```python
from build123d import *
from build123d.topology import SkipClean

# Parameters (mm, degrees)
BOSS_EXTRUDE1_DEPTH    = 3
SKETCH1_R              = 2
BOSS_EXTRUDE1_2_DEPTH  = 3
BOSS_EXTRUDE2_DEPTH    = 3
M4_TAPPED_HOLE1_REACH  = 33.171
M4_TAPPED_HOLE1_BORE_R = 1.65


with BuildPart() as part:
    # Sketch1 → Boss-Extrude1 (new, symmetric)
    with BuildSketch(Plane.XY):
        with BuildLine():
            ThreePointArc((5.5, 0), (0, -5.5), (-5.5, 0))
            Line((-5.5, 0), (-12.42820323, -4))
            ThreePointArc((-12.42820323, -4), (0, -16.42820323), (12.42820323, -4))
            Line((12.42820323, -4), (5.5, 0))
        make_face()
    extrude(amount=BOSS_EXTRUDE1_DEPTH, both=True)



with BuildPart() as body_2:
    # Sketch1 → Boss-Extrude1 2 (new, symmetric)
    with BuildSketch(Plane.XY):
        with BuildLine():
            Line((-3.929058411, 8.75), (-5.402455316, 1.03125))
            ThreePointArc((-5.402455316, 1.03125), (0, 5.5), (5.402455316, 1.03125))
            Line((5.402455316, 1.03125), (3.929058411, 8.75))
            ThreePointArc((3.929058411, 8.75), (0, 12), (-3.929058411, 8.75))
        make_face()
        with Locations((0, 8)):
            Circle(SKETCH1_R, mode=Mode.SUBTRACT)
    extrude(amount=BOSS_EXTRUDE1_2_DEPTH, both=True)


with BuildPart() as part_1:
    with SkipClean():  # the faces are left unmerged after this step: merging them gives an invalid solid
        add(part.part)

        add(body_2.part)  # Boss-Extrude2 merges body 2
        # Sketch1<3> → Boss-Extrude2 (add, symmetric)
        with BuildSketch(Plane.XY):
            with BuildLine():
                ThreePointArc((-3.5, 0), (0, 3.5), (3.5, 0))
                Line((3.5, 0), (5.5, 0))
                ThreePointArc((5.5, 0), (5.475559526, 0.517926522), (5.402455316, 1.03125))
                ThreePointArc((5.402455316, 1.03125), (0, 5.5), (-5.402455316, 1.03125))
                ThreePointArc((-5.402455316, 1.03125), (-5.475559526, 0.517926522), (-5.5, 0))
                Line((-5.5, 0), (-3.5, 0))
            make_face()
            with BuildLine():
                Line((5.5, 0), (3.5, 0))
                ThreePointArc((3.5, 0), (0, -3.5), (-3.5, 0))
                Line((-3.5, 0), (-5.5, 0))
                ThreePointArc((-5.5, 0), (0, -5.5), (5.5, 0))
            make_face()
        extrude(amount=BOSS_EXTRUDE2_DEPTH, both=True)

    # M4 Tapped Hole1 bore → M4 Tapped Hole1 (cut, up to next)
    with BuildSketch(Plane(origin=(0, -16.42820323, 0), x_dir=(-1, 0, 0), z_dir=(0, -1, 0)), mode=Mode.PRIVATE) as m4_tapped_hole1_sk1:
        Circle(M4_TAPPED_HOLE1_BORE_R)
    m4_tapped_hole1_tool1 = extrude(m4_tapped_hole1_sk1.sketch, amount=-M4_TAPPED_HOLE1_REACH, mode=Mode.PRIVATE) & part_1.part
    add(m4_tapped_hole1_tool1.solids().sort_by_distance((0, -16.428203, 0))[0], mode=Mode.SUBTRACT)


solid = part_1.part
```
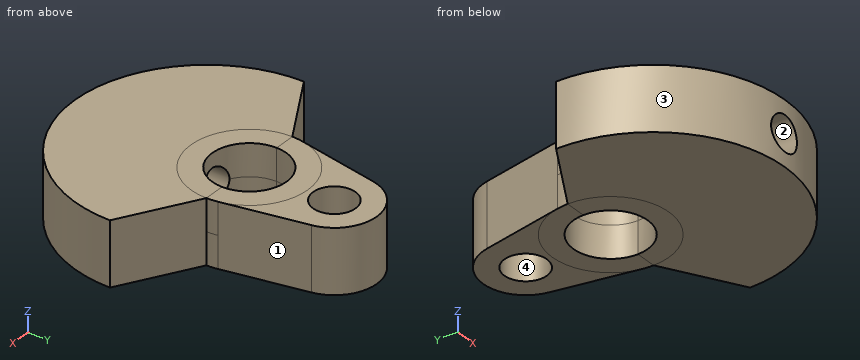
The listing builds one solid part. Answer for the finished solid, in the listing's coordinates (mm). Face numbers are marked on the shaded views. Give positions to 0.01 mm unless a question says otherwise; leave off trailing zeros. Order: outer loops, then holes, each group sorted by start corner. A loop starts at its lowest first (then second) coordinate and runs counter-clockwise, first axis right, second up. Notation, with made-up numbers: M -32.5,51.5 L -14.5,51.5 A30 ccw -14.5,83.5 Z; hole C 14,84 d9. An arc over 180 degrees is marked long. Put each result on its own line as item: value. Start each with the question number.
Item 1: For a pull along Y with two mould halves and no side action, classify the marked faces 1, 2, 3 and 4 as +Y half, -Y half, draft (parallel to the pull), parting line (faces both ways), or undercut.
Item 2: The part is cut by section D-D, the plane y = 8. Determine the outline of the cut face in (x, z).
Item 3: Flat-ended cylindrical pins translate along their axes: P1, Ø1, axis at x = -2, z = -2, coming from the +Y side; P2, Ø3.5, axis at x = 0, y = 8, coming from the -Z side; P3, Ø2, axis at y = -5.5, z = -0.5, coming from the -X side. Find the tip coordinate at first contact, or state that the pin passes through.
Item 4: The part is cut by section B-B, the plane z = -2.5. Determine the outline of the cut face in (x, y), and give its area (3 significant figures).
Item 5: The part is cut by section A-A, the plane x = 0. Determine the outline of the cut face in (y, z), and give its area (3 significant figures).
Item 6: Find the intervals of material crossed by line 1 along Y through (x, z) = (0, -0.4); line 2 along Z through (x, y) = (0, -10.5); line 3 along Y through (x, z) = (-0.75, 1), in increasing order.
Item 7: The part is cut by section C-C, the plane x = 3. Determine the outline of the cut face in (y, z), and give its area (3 significant figures).
Answer key:
1. face 1: +Y half
1. face 2: draft
1. face 3: -Y half
1. face 4: undercut
2. outline: M -4.07,-3 L -2,-3 L -2,3 L -4.07,3 Z; M 2,-3 L 4.07,-3 L 4.07,3 L 2,3 Z
3. P1: stops at y = 11.71
3. P2: passes through
3. P3: stops at x = -12.42
4. outline: M -12.43,-4 A12.43 ccw 12.43,-4 L 5.5,0 A5.5 ccw 5.4,1.03 L 3.93,8.75 A4 ccw -3.93,8.75 L -5.4,1.03 A5.5 ccw -5.5,0 Z; hole C 0,0 d7; hole C 0,8 d4
4. area: 366 mm²
5. outline: M -16.43,-3 L -3.5,-3 L -3.5,-1.65 L -16.43,-1.65 Z; M -16.43,1.65 L -3.5,1.65 L -3.5,3 L -16.43,3 Z; M 3.5,-3 L 6,-3 L 6,3 L 3.5,3 Z; M 10,-3 L 12,-3 L 12,3 L 10,3 Z
5. area: 61.9 mm²
6. line 1: y = 3.5 to 6, 10 to 12
6. line 2: z = -3 to -1.65, 1.65 to 3
6. line 3: y = 3.42 to 6.15, 9.85 to 11.93
7. outline: M -16.06,-3 L -1.8,-3 L -1.8,3 L -16.06,3 Z; M 1.8,-3 L 10.65,-3 L 10.65,3 L 1.8,3 Z
7. area: 139 mm²
